Print and shaded views of the part. All mm, measured from the part's lowest x, y and z. A direction names the side the tool comes from. Coordinates: 2 decimals unless noted, no trailing zeros. Order: outer loops, then holes, each group sorted by start corner. A loop starts at its lowest first (then second) coordinate and runs counter-clockwise, first axis right, second up. Notation, with made-up numbers: (-34, 18) -> (-9, 18) arc R19 cw to (-9, 28) -> close; hole circle Ø2 at (-22.5, 1.25). An arc over 180 degrees is marked (long way). Return JSON: item names as keys, results as strings. Group by question number.
1) Pull direction X, two halves, no side cores. Call the marked faces 3 and 4: +X half, -X half, draft (parallel to the pull), parting line (faces both ways), or undercut.
2) Cut at B-B (y = 4.5). Write the cut outline in (x, z) (1 decimal).
3) Flat gauge pins, fed straight in: pin 1 (0.7 mm diameter, centred on y = 4, z = 7, fed in from +X); pin 2 (2 mm diameter, centred on y = 4.5, z = 11, fed in from -X) (1 decimal); pin 3 (3.5 mm diameter, centred on x = 1, z = 9.5, fed in from +Y) (1 decimal); pin 4 (3 mm diameter, centred on x = 46.32, z = 6.65, fed in from -Y). Where does each tip first touch, or does it go through?
4) Cut at A-A (z = 9). Write the cut outline in (x, y) (1 decimal).
5) Probe line 1 (X direction, y = 3.8, z = 7) (1 decimal); line 2 (X direction, y = 5.35, z = 13.75) (1 decimal); line 3 (X direction, y = 4, z = 5.5) (1 decimal). List the from-to ranges inside material, lowest first.
6) Which spindle directions (+Z, -Z, +X, -X, +Y, -Y) get a long thin tool onto all of the face, cutting with end or side? Do the marked faces 1 and 2. Say none if no direction does.
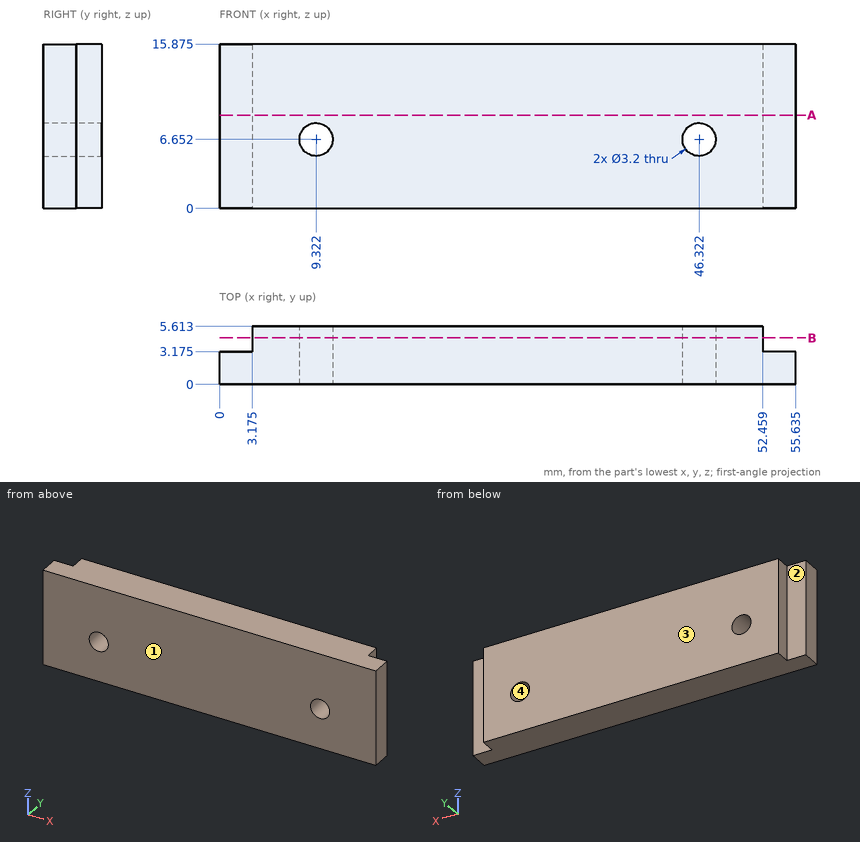
Answers below:
{
 "1": {"face 3": "draft", "face 4": "undercut"},
 "2": {"outline": "(3.2, 0) -> (52.5, 0) -> (52.5, 15.9) -> (3.2, 15.9) -> close; hole circle Ø3.2 at (9.3, 6.7); hole circle Ø3.2 at (46.3, 6.7)"},
 "3": {"pin 1": "stops at x = 52.46", "pin 2": "stops at x = 3.2", "pin 3": "stops at y = 3.2", "pin 4": "passes through"},
 "4": {"outline": "(0, 0) -> (55.6, 0) -> (55.6, 3.2) -> (52.5, 3.2) -> (52.5, 5.6) -> (3.2, 5.6) -> (3.2, 3.2) -> (0, 3.2) -> close"},
 "5": {"line 1": "x = 3.2 to 7.8, 10.9 to 44.8, 47.9 to 52.5", "line 2": "x = 3.2 to 52.5", "line 3": "x = 3.2 to 8.2, 10.4 to 45.2, 47.4 to 52.5"},
 "6": {"face 1": "+Z, -Z, +X, -X, -Y", "face 2": "+Z, -Z, -X, +Y"}
}
